Verification items for the finished model (mm, model axes). Face numbers are marked on the shaded views. A direction names the side the tool comes from. Coordinates: 2 decimals unless noted, no trailing zeros. Write each loop counter-clockwise with the first axis right and the second up, starting at its lowest first coordinate (ties: lowest second). Pieces come first, ordered by that corner, then holes. Notation, with made-up numbers: (39.25, 8) -> (64.25, 8) arc R20 ccw to (64.25, 26) -> close; hole circle Ø7 at (45.5, -36). An arc over 180 degrees is marked (long way). Answer in a Markdown table with one row per item.
```python
from build123d import *

# Parameters (mm, degrees)
BOSS_EXTRUDE1_DEPTH = 6
FILLET1_R           = 6
SKETCH2_R           = 2.5
SKETCH2_R_2         = 0.8
BOSS_EXTRUDE2_DEPTH = 10


with BuildPart() as part:
    # Sketch1 → Boss-Extrude1 (new body)
    with BuildSketch(Plane(origin=(0, 0, 0), x_dir=(1, 0, 0), z_dir=(0, 1, 0))):
        with BuildLine():
            Line((-40.923709509, 2.5), (-29.05, 2.5))
            Line((-29.05, 2.5), (-29.05, 19.525))
            Line((-29.05, 19.525), (-10, 19.525))
            Line((-10, 19.525), (-10, 29.05))
            Line((-10, 29.05), (10, 29.05))
            Line((10, 29.05), (10, 19.525))
            Line((10, 19.525), (29.05, 19.525))
            Line((29.05, 19.525), (29.05, 2.5))
            Line((29.05, 2.5), (40.923709509, 2.5))
            ThreePointArc((40.923709509, 2.5), (0, 41), (-40.923709509, 2.5))
        make_face()
    extrude(amount=BOSS_EXTRUDE1_DEPTH)

    # Fillet1
    fillet1_edges = [part.edges().sort_by_distance(p)[0] for p in [
        (0, 6, -41),
    ]]
    fillet(fillet1_edges, radius=FILLET1_R - 0.0001)  # a hair under: the kernel refuses the full size

    # Sketch2 → Boss-Extrude2 (add)
    # profile 1 of 2: a face of its own
    with BuildSketch(Plane.XZ):
        with Locations(Location((19.05, -25, 0), (0, 0, 270))):
            Circle(SKETCH2_R)
        with Locations(Location((19.05, -25, 0), (0, 0, 270))):
            Circle(SKETCH2_R_2, mode=Mode.SUBTRACT)
    # profile 2 of 2: a face of its own
    with BuildSketch(Plane.XZ):
        with Locations(Location((-19.05, -25, 0), (0, 0, 270))):
            Circle(SKETCH2_R)
        with Locations(Location((-19.05, -25, 0), (0, 0, 270))):
            Circle(SKETCH2_R_2, mode=Mode.SUBTRACT)
    extrude(amount=BOSS_EXTRUDE2_DEPTH)


solid = part.part
```
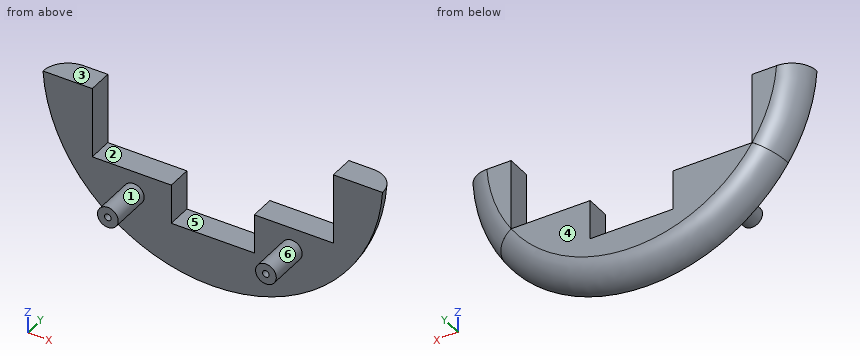
1. Go/stop test with flat-tipped pins: pin 1 (6.5 mm diameter, centred on y = 4.5, z = -8.5, fed in from +X); pin 2 (1.8 mm diameter, centred on x = 4.5, y = 2, fed in from +Z); pin 3 (1.8 mm diameter, centred on y = 1.5, z = -24.5, fed in from -X). Record where each tip stops, or that it passes through.
Findings below:
| item | result |
|---|---|
| pin 1 | stops at x = 40.17 |
| pin 2 | stops at z = -29.05 |
| pin 3 | stops at x = -33.34 |
2. Material ranges on probe 1 along X at (y, z) = (-2.5, -25); probe 2 along Y at (x, z) = (-25, -22); probe 3 along X at (y, z) = (3, -8), recorded low to high. Write a range as from..to.
Findings below:
| item | result |
|---|---|
| probe 1 | x = -21.55..-19.85, -18.25..-16.55, 16.55..18.25, 19.85..21.55 |
| probe 2 | y = 0..6 |
| probe 3 | x = -39.39..-29.05, 29.05..39.39 |
3. Sectioned sample at A-A, the plane y = -1. Record the cut outline in (x, z).
Findings below:
| item | result |
|---|---|
| outline | circle Ø5 at (-19.05, -25); circle Ø5 at (19.05, -25); hole circle Ø1.6 at (-19.05, -25); hole circle Ø1.6 at (19.05, -25) |
4. Release check for a two-part mould opening along X. For the marked faces 4, 5 and 6 record: released by +X, released by -X, zero draft, split by the parting line, or undercut.
Findings below:
| item | result |
|---|---|
| face 4 | zero draft |
| face 5 | undercut |
| face 6 | undercut |
5. Access from +Z, -Z, +X, -X, +Y, -Y to the whole of each face (thin tool, end or side, straight path). Record for the marked faces 1, 2 and 3.
Findings below:
| item | result |
|---|---|
| face 1 | -Y |
| face 2 | +Z, +Y, -Y |
| face 3 | +Z, +X, -X, +Y, -Y |
